Source: CAD feature listing. Evaluate the final solid. Frame: model axes, mm. Face numbers are marked on the shaded views. A direction names the side the tool comes from. Give positions to 0.01 mm unless a question says otherwise; leave off trailing zeros. Loops run counter-clockwise (first coordinate to the right, second up) from the corner with the lowest first, then second, coordinate; pieces in that order, holes last. Notation, with made-up numbers: (69.5, -16) - (107.5, -16) arc R23 ccw to (107.5, 6) - close; hole circle Ø5 at (32.5, 74.5). An arc over 180 degrees is marked (long way). Put each result on its own line as item: value.
```python
from build123d import *

# Parameters (mm, degrees)
F0_R     = 101.6
F1_DEPTH = 6.35
F2_R     = 76.2
F3_DEPTH = 60.325
F4_R     = 101.6
F5_DEPTH = 6.35
F6_R     = 25.4
F7_DEPTH = 73.026


with BuildPart() as f1:
    # F0 (on Right) → F1 (new body)
    with BuildSketch(Plane.YZ):
        Circle(F0_R)
    extrude(amount=F1_DEPTH)

    # F2 (on face) → F3 (join)
    with BuildSketch(Plane.YZ.offset(6.35)):
        Circle(F2_R)
    extrude(amount=F3_DEPTH)

    # F4 (on face) → F5 (join)
    with BuildSketch(Plane.YZ.offset(66.675)):
        Circle(F4_R)
    extrude(amount=F5_DEPTH)

    # F6 (on face) → F7 (cut, through all)
    with BuildSketch(Plane.YZ.offset(73.025)):
        Circle(F6_R)
    extrude(amount=-F7_DEPTH, mode=Mode.SUBTRACT)


solid = f1.part
```
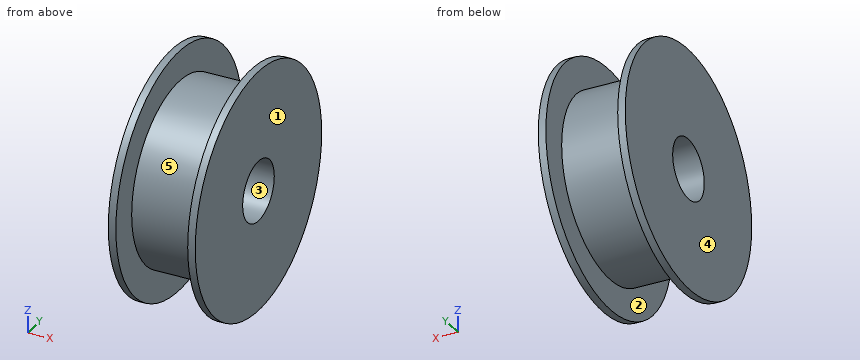
1) Material intervals for line 1 along Z through (x, y) = (38, 0); line 2 along X through (y, z) = (66, -46.5) (3 decimals); line 3 along Y through (x, z) = (39.5, 20), sorted ascending. Write a range as [from, to].
Check result:
line 1: [-76.2, -25.4], [25.4, 76.2]
line 2: [0, 6.35], [66.675, 73.025]
line 3: [-73.53, -15.66], [15.66, 73.53]
2) Access query for the marked faces 4 and 5. Directions: +Z, -Z, +X, -X, +Y, -Y. A direction counts if a zero-diameter tool reaches every point of the face in a straight line with its end or side. Return the directions, or none.
Check result:
face 4: +Z, -Z, -X, +Y, -Y
face 5: none
3) Pin query (flat end, axial travel): P1, Ø6, axis at x = 17.5, z = -54, coming from the +Y side; P2, Ø3, axis at x = 41.5, y = -47.5, coming from the +Z side; P3, Ø4, axis at x = 19.5, y = 39.5, coming from the -Z side. Return the tip coordinate at first contact, or that it passes through.
Check result:
P1: y = 56.62
P2: z = 60.75
P3: z = -66.33
4) Section query C-C, the plane z = -36. Output: boundary loops of the cut face in (x, y) (3 decimals), plus the area to 3 significant figures.
Check result:
outline: (0, -95.008) - (6.35, -95.008) - (6.35, -67.16) - (66.675, -67.16) - (66.675, -95.008) - (73.025, -95.008) - (73.025, 95.008) - (66.675, 95.008) - (66.675, 67.16) - (6.35, 67.16) - (6.35, 95.008) - (0, 95.008) - close
area: 10,500 mm²
5) Section query D-D, the plane y = 63.5. Output: boundary loops of the cut face in (x, z) (3 decimals), plus the area to 3 significant figures.
Check result:
outline: (0, -79.311) - (6.35, -79.311) - (6.35, -42.121) - (66.675, -42.121) - (66.675, -79.311) - (73.025, -79.311) - (73.025, 79.311) - (66.675, 79.311) - (66.675, 42.121) - (6.35, 42.121) - (6.35, 79.311) - (0, 79.311) - close
area: 7,100 mm²
6) Mould query, pull axis X, two halves, no side actions, for the marked faces 1, 2 and 3. Classes: pulls with the +X half, pulls with the -X half, needs draft (parallel to the pull), parting line crosses it, or undercut.
Check result:
face 1: pulls with the +X half
face 2: undercut
face 3: needs draft
7) Section query A-A, the plane z = 0. Output: boundary loops of the cut face in (x, y) (3 decimals).
Check result:
outline: (0, -101.6) - (6.35, -101.6) - (6.35, -76.2) - (66.675, -76.2) - (66.675, -101.6) - (73.025, -101.6) - (73.025, -25.4) - (0, -25.4) - close; (0, 25.4) - (73.025, 25.4) - (73.025, 101.6) - (66.675, 101.6) - (66.675, 76.2) - (6.35, 76.2) - (6.35, 101.6) - (0, 101.6) - close
